Work out the finished part from the listing and answer in its coordinate system (mm). Coordinates: 2 decimals unless noted, no trailing zeros. Write each loop counter-clockwise with the first axis right and the second up, starting at its lowest first coordinate (ties: lowest second). Pieces come first, ordered by that corner, then holes. Notation, with made-up numbers: M 79,30.25 L 95,30.25 A25 cw 95,54.25 Z; hole C 29.25,-12 d5. An arc over 180 degrees is marked long. Answer as CSV lines item,"result". Start each with the question number.
(1) Find the intervals of material crossed by L1, parallel to X at y = 3.25, z = 40; L2, parallel to Z at x = -40, y = 2.5; L3, parallel to X at y = 0.5, z = -1, in increasing order. Write a range as [from, to].
(2) A cutting plane is placed at D-D on z = -23.5. Give the vertices of the cut face in (x, y).
(3) A cutting plane is placed at C-C on z = -40. Give the vertices of the cut face in (x, y).
(4) A cutting plane is placed at A-A on x = 0. Give the vertices of the cut face in (y, z), then the cut area to 3 significant figures.
(5) A cutting plane is placed at B-B on x = -40. Give the vertices of the cut face in (y, z), then the cut area to 3 significant figures.
(6) Flat-ended cylindrical pins translate along their axes: P1, Ø9, axis at x = -59.83, z = -40, coming from the -Y side; P2, Ø7, axis at x = 160.17, z = 0, coming from the -Y side. Find the tip coordinate at first contact, or state that the pin passes through.
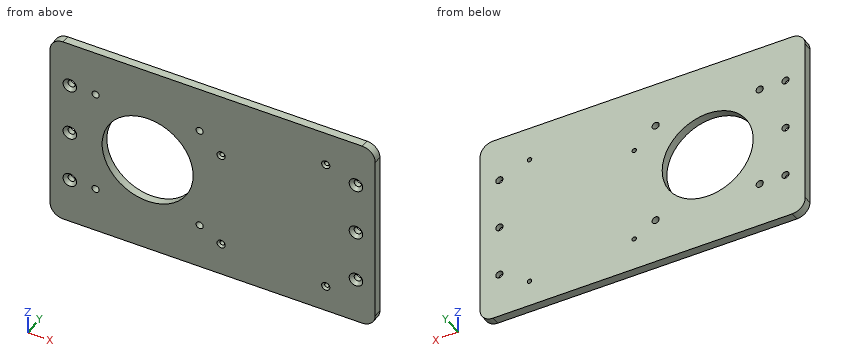
from build123d import *

# Parameters (mm, degrees)
SKETCH1_W                                       = 250
SKETCH1_H                                       = 150
BOSS_EXTRUDE1_DEPTH                             = 6.35
SKETCH2_R                                       = 35
SKETCH2_R_2                                     = 2.75
CUT_EXTRUDE1_DEPTH                              = 7.35
FILLET1_R                                       = 10
CSK_FOR_M5_FLAT_HEAD_MACHINE_SCREW1_D           = 5.5
CSK_FOR_M5_FLAT_HEAD_MACHINE_SCREW1_CSINK_D     = 10.4
CSK_FOR_M5_FLAT_HEAD_MACHINE_SCREW1_CSINK_ANGLE = 90
CSK_FOR_M3_FLAT_HEAD_MACHINE_SCREW1_D           = 3.4
CSK_FOR_M3_FLAT_HEAD_MACHINE_SCREW1_CSINK_D     = 6.3
CSK_FOR_M3_FLAT_HEAD_MACHINE_SCREW1_CSINK_ANGLE = 90


with BuildPart() as part:
    # Sketch1 → Boss-Extrude1 (new body)
    with BuildSketch(Plane(origin=(0, 0, 0), x_dir=(1, 0, 0), z_dir=(0, 1, 0))):
        with Locations((50, 0)):
            Rectangle(SKETCH1_W, SKETCH1_H)
    extrude(amount=BOSS_EXTRUDE1_DEPTH)

    # Sketch2 → Cut-Extrude1 (cut, through all)
    with BuildSketch(Plane(origin=(0, 6.35, 0), x_dir=(1, 0, 0), z_dir=(0, 1, 0))):
        Circle(SKETCH2_R)
        with Locations((-40, 40)):
            Circle(SKETCH2_R_2)
        with Locations((40, 40)):
            Circle(SKETCH2_R_2)
        with Locations((-40, -40)):
            Circle(SKETCH2_R_2)
        with Locations((40, -40)):
            Circle(SKETCH2_R_2)
    extrude(amount=-CUT_EXTRUDE1_DEPTH, mode=Mode.SUBTRACT)

    # Fillet1
    fillet1_edges = [part.edges().sort_by_distance(p)[0] for p in [
        (-75, 3.175, -75),
        (175, 3.175, -75),
        (175, 3.175, 75),
        (-75, 3.175, 75),
    ]]
    fillet(fillet1_edges, radius=FILLET1_R)

    # CSK for M5 Flat Head Machine Screw1 (through all)
    with Locations(Plane(origin=(0, 0, 0), x_dir=(-1, 0, 0), z_dir=(0, -1, 0))):
        with Locations((59.828254494, 40), (59.828254494, 0), (59.828254494, -40), (-160.171745506, 40), (-160.171745506, 0), (-160.171745506, -40)):
            CounterSinkHole(CSK_FOR_M5_FLAT_HEAD_MACHINE_SCREW1_D / 2, CSK_FOR_M5_FLAT_HEAD_MACHINE_SCREW1_CSINK_D / 2, counter_sink_angle=CSK_FOR_M5_FLAT_HEAD_MACHINE_SCREW1_CSINK_ANGLE)

    # CSK for M3 Flat Head Machine Screw1 (through all)
    with Locations(Plane(origin=(0, 0, 0), x_dir=(-1, 0, 0), z_dir=(0, -1, 0))):
        with Locations((-136.964698881, -48.452177006), (-56.504698881, -25.286715777), (-56.504698881, 49.613284223), (-136.964698881, 54.547822994)):
            CounterSinkHole(CSK_FOR_M3_FLAT_HEAD_MACHINE_SCREW1_D / 2, CSK_FOR_M3_FLAT_HEAD_MACHINE_SCREW1_CSINK_D / 2, counter_sink_angle=CSK_FOR_M3_FLAT_HEAD_MACHINE_SCREW1_CSINK_ANGLE)


solid = part.part
Here are the results:
1,L1,"x = [-75, -62.58], [-57.08, -42.75], [-37.25, 37.25], [42.75, 157.42], [162.92, 175]"
1,L2,"z = [-75, -42.75], [-37.25, 37.25], [42.75, 75]"
1,L3,"x = [-75, -64.42], [-55.24, -34.99], [34.99, 155.58], [164.76, 175]"
2,outline,"M -75,0 L -25.94,0 L -25.94,6.35 L -75,6.35 Z; M 25.94,0 L 175,0 L 175,6.35 L 25.94,6.35 Z"
3,outline,"M -75,0 L -65.03,0 L -62.58,2.45 L -62.58,6.35 L -75,6.35 Z; M -57.08,2.45 L -54.63,0 L -42.75,0 L -42.75,6.35 L -57.08,6.35 Z; M -37.25,0 L 37.25,0 L 37.25,6.35 L -37.25,6.35 Z; M 42.75,0 L 154.97,0 L 157.42,2.45 L 157.42,6.35 L 42.75,6.35 Z; M 162.92,2.45 L 165.37,0 L 175,0 L 175,6.35 L 162.92,6.35 Z"
4,outline,"M 0,-75 L 6.35,-75 L 6.35,-35 L 0,-35 Z; M 0,35 L 6.35,35 L 6.35,75 L 0,75 Z"
4,area,"508 mm^2"
5,outline,"M 0,-75 L 6.35,-75 L 6.35,-42.75 L 0,-42.75 Z; M 0,-37.25 L 6.35,-37.25 L 6.35,37.25 L 0,37.25 Z; M 0,42.75 L 6.35,42.75 L 6.35,75 L 0,75 Z"
5,area,"883 mm^2"
6,P1,"stops at y = 0.7"
6,P2,"stops at y = 1.7"
